Geometry check sheet. Reference: the model listing, model coordinates, mm. A direction names the side the tool comes from. Give positions to 0.01 mm unless a question says otherwise; leave off trailing zeros. Loops run counter-clockwise (first coordinate to the right, second up) from the corner with the lowest first, then second, coordinate; pieces in that order, holes last. Notation, with made-up numbers: (-10.75, -16) -> (25.25, -16) arc R25 cw to (25.25, 3) -> close; hole circle Ø7 at (78, -31.5). An arc over 180 degrees is marked (long way). Write each question's results on one line, items separated by ' | '. Start each with the question number.
1) Depth check by flat-ended pin: pin 1 (6 mm diameter, centred on y = -14.5, z = 6, fed in from -X). Enter the tip coordinate at first touch or a pass-through.
2) Draft check along Z on faces 3 (the face through (363.406, -6.419, -6.556)), 4 (the face through (5, -8, -8)), 5 (the face through (5, -9, -6.35)). Enter one of: pulls with the +Z half, pulls with the -Z half, needs draft (parallel to the pull), parting line crosses it, or undercut.
3) Set-up check for faces 1 (the face through (5, -9, 6.35)), 2 (the face through (5, 1.65, 0)): record each of +Z, -Z, +X, -X, +Y, -Y from which the full face is reachable in a straight line by a thin tool's end or side.
4) Sectioned sample at C-C on z = 0.75. Record the cut outline in (x, y) (3 decimals), then the cut area to 3 significant figures.
5) Sectioned sample at B-B on y = -6.5. Record the cut outline in (x, z) (3 decimals), then the cut area to 3 significant figures.
6) Scan lines: line 1 (Z direction, x = 201.5, y = -4.75); line 2 (Y direction, x = 296.5, z = 4); line 3 (X direction, y = -15.25, z = -6.75) (3 decimals). Record each from-to range of solid material in increasing order. Write a range as from..to.
7) Sectioned sample at A-A on x = -101.5. Record the cut outline in (y, z).
```python
from build123d import *

# Parameters (mm, degrees)
BOSS_EXTRUDE1_DEPTH           = 371.475
CUT_RIGHT_SIDE_TOP_DEPTH      = 1
CUT_RIGHT_SIDE_TOP_DEPTH_BACK = 17
CUT_LEFT_SIDE_TOP_DEPTH       = 1
CUT_LEFT_SIDE_TOP_DEPTH_BACK  = 17


with BuildPart() as part:
    # Sketch1 → Boss-Extrude1 (new body, symmetric)
    with BuildSketch(Plane(origin=(0, 0, 0), x_dir=(0, 0, -1), z_dir=(1, 0, 0))):
        Polygon((-6.35, 0), (6.35, 0), (6.35, -17.4), (8, -17.4), (8, 1.65), (-8, 1.65), (-8, -17.4), (-6.35, -17.4), align=None)
    extrude(amount=BOSS_EXTRUDE1_DEPTH, both=True)

    # Sketch7 → Cut-Right-Side-Top (cut, two sides)
    with BuildSketch(Plane(origin=(0, 0, -8), x_dir=(-1, 0, 0), z_dir=(0, 0, -1))) as cut_right_side_top_sk:
        Polygon((-371.475, 1.65), (-352.425, -17.4), (-371.475, -17.4), align=None)
    extrude(amount=CUT_RIGHT_SIDE_TOP_DEPTH, mode=Mode.SUBTRACT)
    extrude(cut_right_side_top_sk.sketch, amount=-CUT_RIGHT_SIDE_TOP_DEPTH_BACK, mode=Mode.SUBTRACT)

    # Sketch5 → Cut-Left-Side-Top (cut, two sides)
    with BuildSketch(Plane(origin=(0, 0, -8), x_dir=(-1, 0, 0), z_dir=(0, 0, -1))) as cut_left_side_top_sk:
        Polygon((371.475, 1.65), (352.425, -17.4), (371.475, -17.4), align=None)
    extrude(amount=CUT_LEFT_SIDE_TOP_DEPTH, mode=Mode.SUBTRACT)
    extrude(cut_left_side_top_sk.sketch, amount=-CUT_LEFT_SIDE_TOP_DEPTH_BACK, mode=Mode.SUBTRACT)


solid = part.part
```
Result:
1) pin 1: x = -358.3
2) face 3: needs draft | face 4: pulls with the -Z half | face 5: undercut
3) face 1: +X, -X, -Y | face 2: +Z, -Z, +X, -X, +Y
4) outline: (-371.475, 1.65) -> (-369.825, 0) -> (369.825, 0) -> (371.475, 1.65) -> close | area: 1,220 mm^2
5) outline: (-363.325, -8) -> (363.325, -8) -> (363.325, -6.35) -> (-363.325, -6.35) -> close; (-363.325, 6.35) -> (363.325, 6.35) -> (363.325, 8) -> (-363.325, 8) -> close | area: 2,400 mm^2
6) line 1: -8..-6.35, 6.35..8 | line 2: 0..1.65 | line 3: -354.575..354.575
7) outline: (-17.4, -8) -> (1.65, -8) -> (1.65, 8) -> (-17.4, 8) -> (-17.4, 6.35) -> (0, 6.35) -> (0, -6.35) -> (-17.4, -6.35) -> close
